Here's how the part is built. I have some questions about the finished solid (model axes, mm). Give positions to 0.01 mm unless a question says otherwise; leave off trailing zeros. Write each loop counter-clockwise with the first axis right and the second up, starting at its lowest first coordinate (ties: lowest second). Pieces come first, ordered by that corner, then holes. Notation, with made-up numbers: (65.5, 35.5) -> (77.5, 35.5) arc R29 ccw to (77.5, 73.5) -> close; hole circle Ø8 at (15, 35.25). An arc over 180 degrees is marked (long way). Use CSV: the item, a comma, the result in double quotes. Start each with the question number.
(1) For pin 1 Ø12 at (x, y) = (-9, 13) entering from -Z; pin 2 Ø1.6 at (x, y) = (19.5, -18.5) entering from -Z, each with a flat end and sliding along its axis, tell me the tip position at first contact or that it passes through.
(2) Suppose I cut it at D-D on y = 26.5. List the corners of the cut face in (x, z) for me, plus the area to 3 significant figures.
(3) I need wall thicknesses on L1, parallel to Y at x = 19, z = 3.65; L2, parallel to Y at x = -21.5, z = 0.4; L3, parallel to Y at x = -25, z = 4.3. Which ranges of each line are inside material? Lowest first, please. Write a range as [from, to].
(4) Suppose I cut it at C-C on y = 19.5. List the corners of the cut face in (x, z) for me, plus the area to 3 significant figures.
(5) Suppose I cut it at A-A on x = 19. List the corners of the cut face in (y, z) for me.
(6) Suppose I cut it at B-B on z = 1.25. List the corners of the cut face in (x, y) for me.
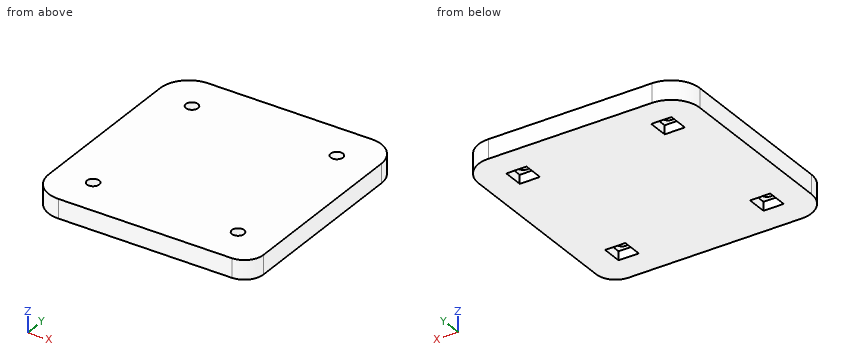
from build123d import *

# Parameters (mm, degrees)
F0_W     = 5.3
F0_H     = 5.3
F0_R     = 1.6
F1_DEPTH = 5
F2_DEPTH = 2.3


with BuildPart() as f1:
    # F0 (on Top) → F1 (new body)
    with BuildSketch(Plane.XY):
        with BuildLine():
            ThreePointArc((29, 22), (26.803301, 27.303301), (21.5, 29.5))
            Line((21.5, 29.5), (-21.5, 29.5))
            ThreePointArc((-21.5, 29.5), (-26.803301, 27.303301), (-29, 22))
            Line((-29, 22), (-29, -22))
            ThreePointArc((-29, -22), (-26.803301, -27.303301), (-21.5, -29.5))
            Line((-21.5, -29.5), (24, -29.5))
            ThreePointArc((24, -29.5), (27.535534, -28.035534), (29, -24.5))
            Line((29, -24.5), (29, 22))
        make_face()
        with Locations((-19, -19.5)):
            Rectangle(F0_W, F0_H, mode=Mode.SUBTRACT)
        with Locations((19, -19.5)):
            Rectangle(F0_W, F0_H, mode=Mode.SUBTRACT)
        with Locations((-19, 19.5)):
            Rectangle(F0_W, F0_H, mode=Mode.SUBTRACT)
        with Locations((19, 19.5)):
            Rectangle(F0_W, F0_H, mode=Mode.SUBTRACT)
        with Locations((-19, 19.5)):
            Rectangle(F0_W, F0_H)
        with Locations((-19, 19.5)):
            Circle(F0_R, mode=Mode.SUBTRACT)
        with Locations((19, 19.5)):
            Rectangle(F0_W, F0_H)
        with Locations((19, 19.5)):
            Circle(F0_R, mode=Mode.SUBTRACT)
        with Locations((19, -19.5)):
            Rectangle(F0_W, F0_H)
        with Locations((19, -19.5)):
            Circle(F0_R, mode=Mode.SUBTRACT)
        with Locations((-19, -19.5)):
            Rectangle(F0_W, F0_H)
        with Locations((-19, -19.5)):
            Circle(F0_R, mode=Mode.SUBTRACT)
    extrude(amount=F1_DEPTH)

    # F0 (on Top) → F2 (cut)
    with BuildSketch(Plane.XY):
        with Locations((-19, 19.5)):
            Rectangle(F0_W, F0_H)
        with Locations((-19, 19.5)):
            Circle(F0_R, mode=Mode.SUBTRACT)
        with Locations((19, 19.5)):
            Rectangle(F0_W, F0_H)
        with Locations((19, 19.5)):
            Circle(F0_R, mode=Mode.SUBTRACT)
        with Locations((-19, -19.5)):
            Rectangle(F0_W, F0_H)
        with Locations((-19, -19.5)):
            Circle(F0_R, mode=Mode.SUBTRACT)
        with Locations((19, -19.5)):
            Rectangle(F0_W, F0_H)
        with Locations((19, -19.5)):
            Circle(F0_R, mode=Mode.SUBTRACT)
    extrude(amount=F2_DEPTH, mode=Mode.SUBTRACT)


solid = f1.part
Geometry says:
1,pin 1,"z = 0"
1,pin 2,"z = 2.3"
2,outline,"(-27.5, 0) -> (27.5, 0) -> (27.5, 5) -> (-27.5, 5) -> close"
2,area,"275 mm²"
3,L1,"[-29.5, -21.1], [-17.9, 17.9], [21.1, 29.5]"
3,L2,"[-29.5, -22.15], [-16.85, 16.85], [22.15, 29.5]"
3,L3,"[-28.63, 28.63]"
4,outline,"(-29, 0) -> (-21.65, 0) -> (-21.65, 2.3) -> (-20.6, 2.3) -> (-20.6, 5) -> (-29, 5) -> close; (-17.4, 2.3) -> (-16.35, 2.3) -> (-16.35, 0) -> (16.35, 0) -> (16.35, 2.3) -> (17.4, 2.3) -> (17.4, 5) -> (-17.4, 5) -> close; (20.6, 2.3) -> (21.65, 2.3) -> (21.65, 0) -> (29, 0) -> (29, 5) -> (20.6, 5) -> close"
4,area,"248 mm²"
5,outline,"(-29.5, 0) -> (-22.15, 0) -> (-22.15, 2.3) -> (-21.1, 2.3) -> (-21.1, 5) -> (-29.5, 5) -> close; (-17.9, 2.3) -> (-16.85, 2.3) -> (-16.85, 0) -> (16.85, 0) -> (16.85, 2.3) -> (17.9, 2.3) -> (17.9, 5) -> (-17.9, 5) -> close; (21.1, 2.3) -> (22.15, 2.3) -> (22.15, 0) -> (29.5, 0) -> (29.5, 5) -> (21.1, 5) -> close"
6,outline,"(-29, -22) arc R7.5 ccw to (-21.5, -29.5) -> (24, -29.5) arc R5 ccw to (29, -24.5) -> (29, 22) arc R7.5 ccw to (21.5, 29.5) -> (-21.5, 29.5) arc R7.5 ccw to (-29, 22) -> close; hole (-21.65, -22.15) -> (-16.35, -22.15) -> (-16.35, -16.85) -> (-21.65, -16.85) -> close; hole (-21.65, 16.85) -> (-16.35, 16.85) -> (-16.35, 22.15) -> (-21.65, 22.15) -> close; hole (16.35, -22.15) -> (21.65, -22.15) -> (21.65, -16.85) -> (16.35, -16.85) -> close; hole (16.35, 16.85) -> (21.65, 16.85) -> (21.65, 22.15) -> (16.35, 22.15) -> close"
